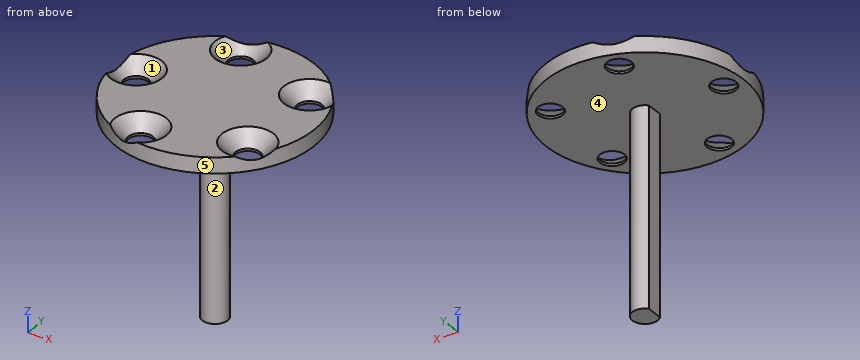
Autodesk Inventor part; units mm, degrees
ref_plane "YZ Plane" through (0, 0, 0) normal (1, 0, 0) x (0, 1, 0)
ref_plane "XZ Plane" through (0, 0, 0) normal (0, 1, 0) x (-1, 0, 0)
ref_plane "XY Plane" through (0, 0, 0) normal (0, 0, 1) x (1, 0, 0)
ref_plane "Work Plane1" through (14.6215, -13.2895, -4.736) normal (0, 0, 1) x (1, 0, 0)
sketch "Sketch1" plane through (14.6215, -13.2895, -4.736) normal (0, 0, 1) x (1, 0, 0)
  circle A0 centre (0, 0) radius 4
  arc A1 (-1.3, -1.0954) -> (-1.3, 1.0954) centre (0, 0) ccw
  line L0 (-1.3, -1.0954) -> (-1.3, 1.0954)
  circle A2 centre (0, 0) radius 6
  circle A3 centre (0, 0) radius 12.5
  circle A4 centre (0, 0) radius 1.3331
  point P0 (-14.6215, 13.2895)
  dimension "d0" = 12
  dimension "d1" = 25
extrude "Extrusion1" add sketch "Sketch1" along normal blind 2 contours A0 | L0 A4 A1 | A4 L0 | L0 A4 | A2 | A3
sketch "Sketch2" plane through (14.6215, -13.2895, -4.736) normal (0, 0, 1) x (1, 0, 0)
  circle A0 centre (0, 0) radius 4
  arc A1 (-1.3, -1.0954) -> (-1.3, 1.0954) centre (0, 0) ccw
  line L0 (-1.3, -1.0954) -> (-1.3, 1.0954)
  circle A2 centre (0, 0) radius 6
  circle A3 centre (0, 0) radius 12.5
  circle A4 centre (-10, 0) radius 1.55
  circle A5 centre (-3.0902, -9.5106) radius 1.55
  circle A6 centre (8.0902, -5.8779) radius 1.55
  circle A7 centre (8.0902, 5.8779) radius 1.55
  circle A8 centre (-3.0902, 9.5106) radius 1.55
  point P0 (-14.6215, 13.2895)
  dimension "d4" = 12
  dimension "d5" = 25
  dimension "d6" = 3.1
  dimension "d7" = 10
  dimension "d10" = 360
extrude "Extrusion2" cut sketch "Sketch2" along normal blind 22 contours A4 | A5 | A6 | A7 | A8
chamfer "Chamfer1" distance 1.7 angle 45 5 edges at (9.9813, -3.779, -2.736) (3.0715, -13.2895, -2.736) (21.1616, -7.4117, -2.736) (21.1616, -19.1674, -2.736) (9.9813, -22.8001, -2.736)
sketch "Sketch3" plane through (14.6215, -13.2895, -4.736) normal (0, 0, -1) x (-1, 0, 0)
  circle A0 centre (0, 0) radius 1.6
  line L0 (1.2, -1.0583) -> (1.2, 1.0583)
  point P0 (14.6215, 13.2895)
  point P1 (0.6764, 1.45)
  point P2 (-0.6764, 1.45)
  dimension "d17" = 3.2
  dimension "d21" = 1.2
extrude "Extrusion3" add sketch "Sketch3" along normal blind 25 contours L0 A0 picked at (0.2667, 0)
properties part number "formadol"
Read the model definition and answer for the solid it produces. Units are mm, in the model's axes. Face numbers are marked on the shaded views. A direction names the side the tool comes from. Coordinates: 2 decimals unless noted, no trailing zeros. Loops run counter-clockwise (first coordinate to the right, second up) from the corner with the lowest first, then second, coordinate; pieces in that order, holes last. Notation, with made-up numbers: (61, -12.5) -> (66, -12.5) arc R24 cw to (66, 3.5) -> close; hole circle Ø2 at (11.25, -27). An arc over 180 degrees is marked (long way). Answer in a Markdown table with one row per item.
Item 1: A cutting plane is placed at A-A on z = -8. Determine the outline of the cut face in (x, y).
Returned:
| item | result |
|---|---|
| outline | (13.42, -14.35) arc R1.6 ccw (long way) to (13.42, -12.23) -> close |
Item 2: A cutting plane is placed at B-B on x = 12.25. Give the number of separate pieces and of enclosed holes in the cut face, plus the area to 3 significant figures.
Returned:
| item | result |
|---|---|
| separate pieces | 3 |
| enclosed holes | 0 |
| area | 32.1 mm^2 |
Item 3: For a pull along X with two mould halves and no side action, classify the marked faces 3, 4 and 5 as released by +X, released by -X, zero draft, split by the parting line, or undercut.
Returned:
| item | result |
|---|---|
| face 3 | undercut |
| face 4 | zero draft |
| face 5 | split by the parting line |
Item 4: For the marked faces 1 and 2, determine the directions among +Z, -Z, +X, -X, +Y, -Y from which every point of the face is accessible in a straight line to the end or side of a thin tool.
Returned:
| item | result |
|---|---|
| face 1 | +Z |
| face 2 | -Z |
Item 5: Straight lines are drawn through the part: line 1 along Z through (x, y) = (16.5, -23.25); line 2 along Y through (x, z) = (14.25, -12); line 3 along Z through (x, y) = (13, -20.75). For each, find the intervals that lie inside material, in ascending order. Write a range as [from, to].
Returned:
| item | result |
|---|---|
| line 1 | z = [-4.74, -2.74] |
| line 2 | y = [-14.85, -11.73] |
| line 3 | z = [-4.74, -3.46] |
Item 6: Each of these flat-tipped pins is pushed along its axis until it touches: P1, Ø4, axis at y = -16.5, z = -10.5, coming from the +X side; P2, Ø10, axis at y = -20.5, z = -25, coming from the -X side; P3, Ø2.5, axis at y = -13.5, z = -12.5, coming from the -X side; P4, Ø5, axis at x = 6.5, y = -4, coming from the -Z side. Where does it stop, or does it pass through?
Returned:
| item | result |
|---|---|
| P1 | stops at x = 15.67 |
| P2 | passes through |
| P3 | stops at x = 13.42 |
| P4 | stops at z = -4.74 |
